from build123d import *

# Parameters (mm, degrees)
SKETCH1_W               = 127
SKETCH1_H               = 279.4
BOSS_EXTRUDE1_DEPTH     = 9.525
SKETCH2_W               = 9.525
SKETCH2_H               = 25.4
BOSS_EXTRUDE2_DEPTH     = 9.525
LPATTERN1_COUNT         = 6
LPATTERN1_PITCH         = 50.8
MIRROR1_COPY_1_SKETCH_W = 9.525
MIRROR1_COPY_1_SKETCH_H = 25.4
MIRROR1_COPY_1_DEPTH    = 9.525
MIRROR1_COPY_2_SKETCH_W = 9.525
MIRROR1_COPY_2_SKETCH_H = 25.4
MIRROR1_COPY_2_DEPTH    = 9.525
MIRROR1_COPY_3_SKETCH_W = 9.525
MIRROR1_COPY_3_SKETCH_H = 25.4
MIRROR1_COPY_3_DEPTH    = 9.525
MIRROR1_COPY_4_SKETCH_W = 9.525
MIRROR1_COPY_4_SKETCH_H = 25.4
MIRROR1_COPY_4_DEPTH    = 9.525
MIRROR1_COPY_5_SKETCH_W = 9.525
MIRROR1_COPY_5_SKETCH_H = 25.4
MIRROR1_COPY_5_DEPTH    = 9.525
SKETCH3_W               = 9.525
SKETCH3_H               = 25.4
BOSS_EXTRUDE3_DEPTH     = 9.525
LPATTERN2_COUNT         = 2
LPATTERN2_PITCH         = 50.8
SKETCH4_W               = 20.32
SKETCH4_H               = 203.2
CUT_EXTRUDE1_DEPTH      = 9.525


with BuildPart() as part:
    # Sketch1 → Boss-Extrude1 (new body)
    with BuildSketch(Plane(origin=(0, 0, 0), x_dir=(0, 0, -1), z_dir=(1, 0, 0))):
        Rectangle(SKETCH1_W, SKETCH1_H)
    extrude(amount=BOSS_EXTRUDE1_DEPTH)

    # Sketch2 → Boss-Extrude2 (add)
    with BuildSketch(Plane.XY.offset(63.5)):
        with Locations((4.7625, 127)):
            Rectangle(SKETCH2_W, SKETCH2_H)
    boss_extrude2 = extrude(amount=BOSS_EXTRUDE2_DEPTH)

    # LPattern1: Boss-Extrude2 ×6
    with Locations(*[(0, -i * LPATTERN1_PITCH, 0) for i in range(1, LPATTERN1_COUNT)]):
        add(boss_extrude2)

    # Mirror1: Boss-Extrude2 across plane
    add(boss_extrude2.mirror(Plane.XY))

    # Mirror1 copy 1 sketch → Mirror1 copy 1 (add)
    with BuildSketch(Plane(origin=(0, -50.8, -63.5), x_dir=(1, 0, 0), z_dir=(0, 0, -1))):
        with Locations((4.7625, -127)):
            Rectangle(MIRROR1_COPY_1_SKETCH_W, MIRROR1_COPY_1_SKETCH_H)
    extrude(amount=MIRROR1_COPY_1_DEPTH)

    # Mirror1 copy 2 sketch → Mirror1 copy 2 (add)
    with BuildSketch(Plane(origin=(0, -101.6, -63.5), x_dir=(1, 0, 0), z_dir=(0, 0, -1))):
        with Locations((4.7625, -127)):
            Rectangle(MIRROR1_COPY_2_SKETCH_W, MIRROR1_COPY_2_SKETCH_H)
    extrude(amount=MIRROR1_COPY_2_DEPTH)

    # Mirror1 copy 3 sketch → Mirror1 copy 3 (add)
    with BuildSketch(Plane(origin=(0, -152.4, -63.5), x_dir=(1, 0, 0), z_dir=(0, 0, -1))):
        with Locations((4.7625, -127)):
            Rectangle(MIRROR1_COPY_3_SKETCH_W, MIRROR1_COPY_3_SKETCH_H)
    extrude(amount=MIRROR1_COPY_3_DEPTH)

    # Mirror1 copy 4 sketch → Mirror1 copy 4 (add)
    with BuildSketch(Plane(origin=(0, -203.2, -63.5), x_dir=(1, 0, 0), z_dir=(0, 0, -1))):
        with Locations((4.7625, -127)):
            Rectangle(MIRROR1_COPY_4_SKETCH_W, MIRROR1_COPY_4_SKETCH_H)
    extrude(amount=MIRROR1_COPY_4_DEPTH)

    # Mirror1 copy 5 sketch → Mirror1 copy 5 (add)
    with BuildSketch(Plane(origin=(0, -254, -63.5), x_dir=(1, 0, 0), z_dir=(0, 0, -1))):
        with Locations((4.7625, -127)):
            Rectangle(MIRROR1_COPY_5_SKETCH_W, MIRROR1_COPY_5_SKETCH_H)
    extrude(amount=MIRROR1_COPY_5_DEPTH)

    # Sketch3 → Boss-Extrude3 (add)
    with BuildSketch(Plane.XZ.offset(139.7)):
        with Locations((4.7625, 25.4)):
            Rectangle(SKETCH3_W, SKETCH3_H)
    boss_extrude3 = extrude(amount=BOSS_EXTRUDE3_DEPTH)

    # LPattern2: Boss-Extrude3 ×2
    with Locations(*[(0, 0, -i * LPATTERN2_PITCH) for i in range(1, LPATTERN2_COUNT)]):
        add(boss_extrude3)

    # Sketch4 → Cut-Extrude1 (cut)
    with BuildSketch(Plane(origin=(9.525, 0, 0), x_dir=(0, 0, -1), z_dir=(1, 0, 0))):
        with Locations((-34.29, -12.7)):
            Rectangle(SKETCH4_W, SKETCH4_H)
    cut_extrude1 = extrude(amount=-CUT_EXTRUDE1_DEPTH, mode=Mode.SUBTRACT)

    # Mirror2: Cut-Extrude1 across plane
    add(cut_extrude1.mirror(Plane.XY), mode=Mode.SUBTRACT)


solid = part.part
The model under review builds one solid part; all positions refer to its coordinate system, in mm. A direction names the side the tool comes from. Round coordinates to 2 decimals unless told otherwise and drop trailing zeros. Write each loop counter-clockwise with the first axis right and the second up, starting at its lowest first coordinate (ties: lowest second). Pieces come first, ordered by that corner, then holes. Notation, with made-up numbers: M 41.25,35 L 68.25,35 A26 ccw 68.25,71 Z; hole C 19,89.5 d5. An arc over 180 degrees is marked long. Use a Markdown table: item, result. Add a question column.
Q1. Insertion check: pin 1 (5 mm diameter, centred on x = 6.5, y = -4.5, fed in from +Z); pin 2 (5 mm diameter, centred on x = 3.5, y = -41.5, fed in from -Z). Each pin has a flat end and moves straight along its axis. Give the tip position at first contact, or say it passes through.
Q2. To check wall thickness, follow line 1 (Z direction, x = 9.25, y = 78.5) (3 decimals); line 2 (Z direction, x = 3.5, y = 8); line 3 (Y direction, x = 5, z = -37.5) (3 decimals). State the ranges of each line that lie inside material, in increasing order.
Q3. Machinability: for faces 1 (the face through (5, -144, 12.7)), 2 (the face through (5, 101, -63.5)), 3 (the face through (5, -149.225, 26)), 4 (the face through (5, 51, 63.5)), 5 (the face through (5, -127, -73.025)), which of the approach directions +Z, -Z, +X, -X, +Y, -Y give a long, thin tool a straight path to every point of the face, cutting with its end or side? Answer none if there is none.
Q4. The part is to be moulded in two halves that separate along Z. For faces 6 (the face through (5, -14, 44.45)), 7 (the face through (5, 38.1, 68)), 8 (the face through (5, 76, -73.025)), say which applies: pulls with the +Z half, pulls with the -Z half, needs draft (parallel to the pull), parting line crosses it, or undercut.
Q5. We need section D-D, the plane z = 3. State the section outline as (x, y) points (3 decimals).
Q6. We need section B-B, the plane x = 7.25. Count the separate pieces of the cut face and the enclosed holes in it, plus the area to 3 significant figures.
Q7. We need section A-A, the plane y = -2.5. State the section outline as (x, z) points (3 decimals).
Q8. We need section C-C, the plane y = -73. State the section outline as (x, z) points (3 decimals).
Findings below:
| question | item | result |
|---|---|---|
| 1 | pin 1 | stops at z = 63.5 |
| 1 | pin 2 | stops at z = -63.5 |
| 2 | line 1 | z = -73.025 to -44.45, -24.13 to 24.13, 44.45 to 73.025 |
| 2 | line 2 | z = -63.5 to -44.45, -24.13 to 24.13, 44.45 to 63.5 |
| 2 | line 3 | y = -149.225 to -114.3, 88.9 to 139.7 |
| 3 | face 1 | +X, -X, -Y |
| 3 | face 2 | -Z, +X, -X |
| 3 | face 3 | +Z, -Z, +X, -X, -Y |
| 3 | face 4 | +Z, +X, -X |
| 3 | face 5 | -Z, +X, -X, +Y, -Y |
| 4 | face 6 | undercut |
| 4 | face 7 | needs draft |
| 4 | face 8 | pulls with the -Z half |
| 5 | outline | M 0,-139.7 L 9.525,-139.7 L 9.525,139.7 L 0,139.7 Z |
| 6 | separate pieces | 1 |
| 6 | enclosed holes | 2 |
| 6 | area | 30,600 mm² |
| 7 | outline | M 0,-63.5 L 9.525,-63.5 L 9.525,-44.45 L 0,-44.45 Z; M 0,-24.13 L 9.525,-24.13 L 9.525,24.13 L 0,24.13 Z; M 0,44.45 L 9.525,44.45 L 9.525,63.5 L 0,63.5 Z |
| 8 | outline | M 0,-73.025 L 9.525,-73.025 L 9.525,-44.45 L 0,-44.45 Z; M 0,-24.13 L 9.525,-24.13 L 9.525,24.13 L 0,24.13 Z; M 0,44.45 L 9.525,44.45 L 9.525,73.025 L 0,73.025 Z |
